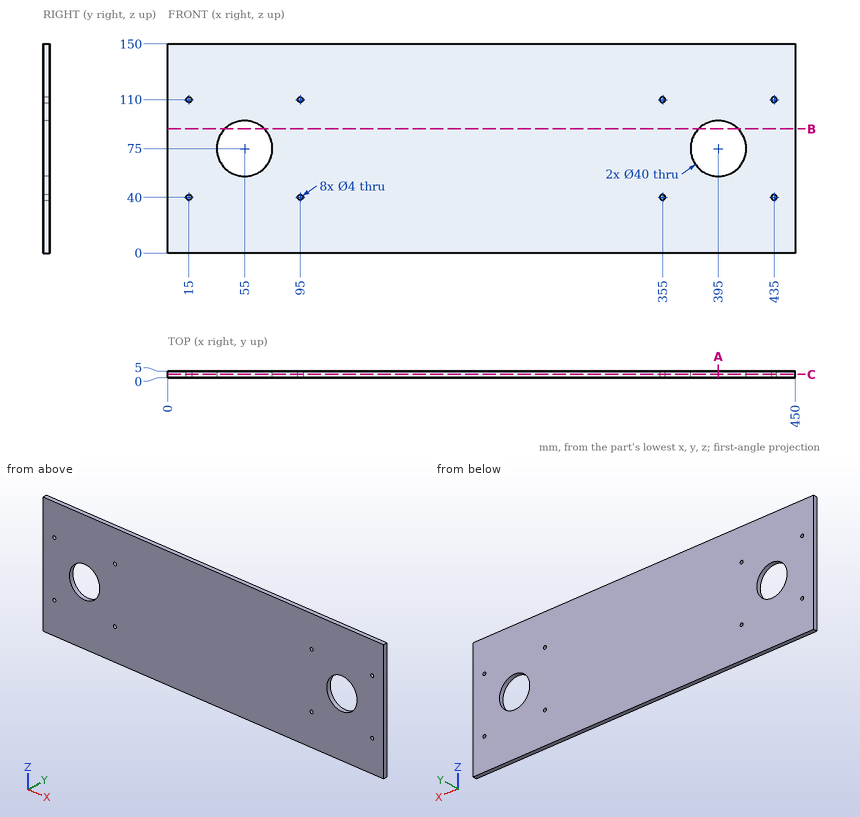
Here's the drawing with two shaded views (mm, measured from the low corner). I have some questions. Round coordinates to 2 decimals unless told otherwise and drop trailing zeros. Write each loop counter-clockwise with the first axis right and the second up, starting at its lowest first coordinate (ties: lowest second). Pieces come first, ordered by that corner, then holes.
(1) Suppose I cut it at C-C on y = 2.6. State how many separate pieces and enclosed holes the cut face has, and give its area (3 significant figures).
Findings below:
separate pieces: 1
enclosed holes: 10
area: 64,900 mm2
(2) For pin 1 (3.5 mm diameter, centred on x = 95, z = 110, fed in from +Y), with a flat end and sliding along its axis, tell me the tip position at first contact or that it passes through.
Findings below:
pin 1: passes through
(3) If I drill on probe 1 along X at (y, z) = (1.45, 40); probe 2 along Z at (x, y) = (15, 2.1); probe 3 along Z at (x, y) = (395, 2), over which ranges is the centre line in solid material (lowest first)?
Findings below:
probe 1: x = 0 to 13, 17 to 93, 97 to 353, 357 to 433, 437 to 450
probe 2: z = 0 to 38, 42 to 108, 112 to 150
probe 3: z = 0 to 55, 95 to 150
(4) Suppose I cut it at B-B on z = 89. Write out the boundary of the cut face in (x, y).
Findings below:
outline: (0, 0) - (40.72, 0) - (40.72, 5) - (0, 5) - close; (69.28, 0) - (380.72, 0) - (380.72, 5) - (69.28, 5) - close; (409.28, 0) - (450, 0) - (450, 5) - (409.28, 5) - close
(5) Suppose I cut it at A-A on x = 395. Write out the boundary of the cut face in (y, z), and give its area (3 significant figures).
Findings below:
outline: (0, 0) - (5, 0) - (5, 55) - (0, 55) - close; (0, 95) - (5, 95) - (5, 150) - (0, 150) - close
area: 550 mm2
